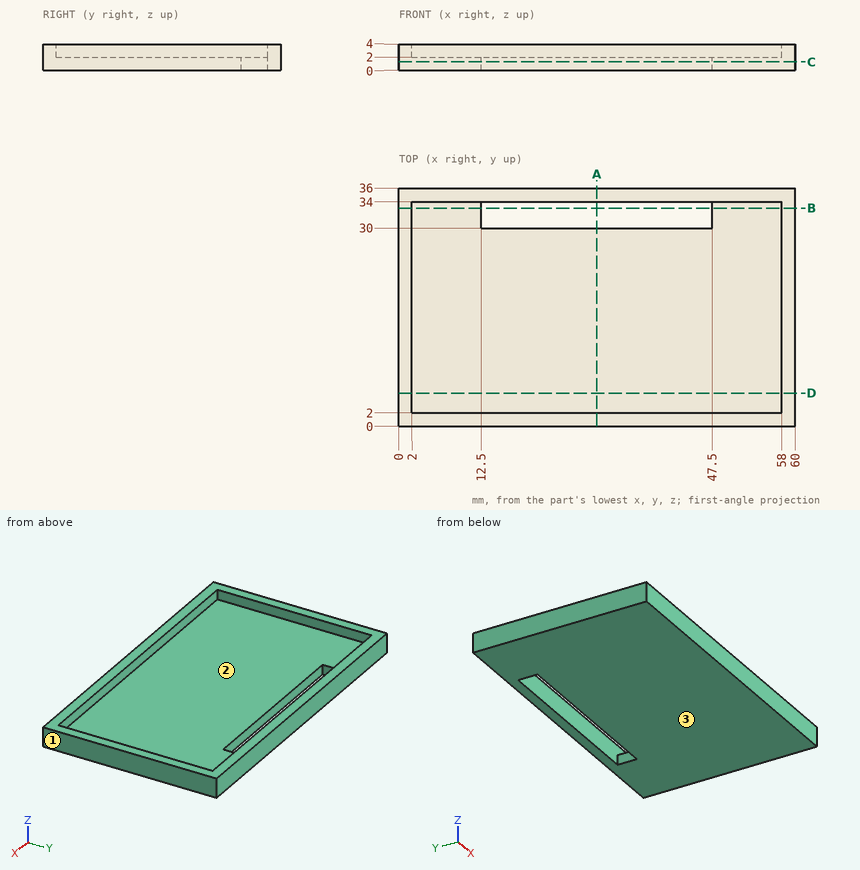
Geometry check sheet. Reference: drawing and pictorial views, mm from the part's lowest x, y, z. Coordinates: 2 decimals unless noted, no trailing zeros. Order: outer loops, then holes, each group sorted by start corner. A loop starts at its lowest first (then second) coordinate and runs counter-clockwise, first axis right, second up.
Item 1: Section check A-A (x = 30). Enter the section's corners in (y, z).
Item 2: Section check C-C (z = 1.3). Enter the section's corners in (x, y), plus the area to 3 significant figures.
Item 3: Scan lines: line 1 along Y through (x, z) = (42.5, 3.7); line 2 along X through (y, z) = (15, 3.35); line 3 along Y through (x, z) = (39.5, 1.1). Record each from-to range of solid material in increasing order.
Item 4: Depth check by flat-ended pin: pin 1 (9.5 mm diameter, centred on x = 42, y = 26, fed in from +Z). Enter the tip coordinate at first touch or a pass-through.
Item 5: Section check D-D (y = 5). Enter the section's corners in (x, z), plus the area to 3 significant figures.
Item 6: Mould release check, pull along X, two halves, no side actions. Record for the marked faces 1, 2 and 3: released by +X, released by -X, zero draft, split by the parting line, or undercut.
Item 7: Section check B-B (y = 33). Enter the section's corners in (x, z), plus the area to 3 significant figures.
Check sheet entries:
1. outline: (0, 0) - (30, 0) - (30, 2) - (2, 2) - (2, 4) - (0, 4) - close; (34, 0) - (36, 0) - (36, 4) - (34, 4) - close
2. outline: (0, 0) - (60, 0) - (60, 36) - (0, 36) - close; hole (12.5, 30) - (47.5, 30) - (47.5, 34) - (12.5, 34) - close
2. area: 2,020 mm2
3. line 1: y = 0 to 2, 34 to 36
3. line 2: x = 0 to 2, 58 to 60
3. line 3: y = 0 to 30, 34 to 36
4. pin 1: stops at z = 2
5. outline: (0, 0) - (60, 0) - (60, 4) - (58, 4) - (58, 2) - (2, 2) - (2, 4) - (0, 4) - close
5. area: 128 mm2
6. face 1: released by +X
6. face 2: undercut
6. face 3: zero draft
7. outline: (0, 0) - (12.5, 0) - (12.5, 2) - (2, 2) - (2, 4) - (0, 4) - close; (47.5, 0) - (60, 0) - (60, 4) - (58, 4) - (58, 2) - (47.5, 2) - close
7. area: 58.0 mm2
